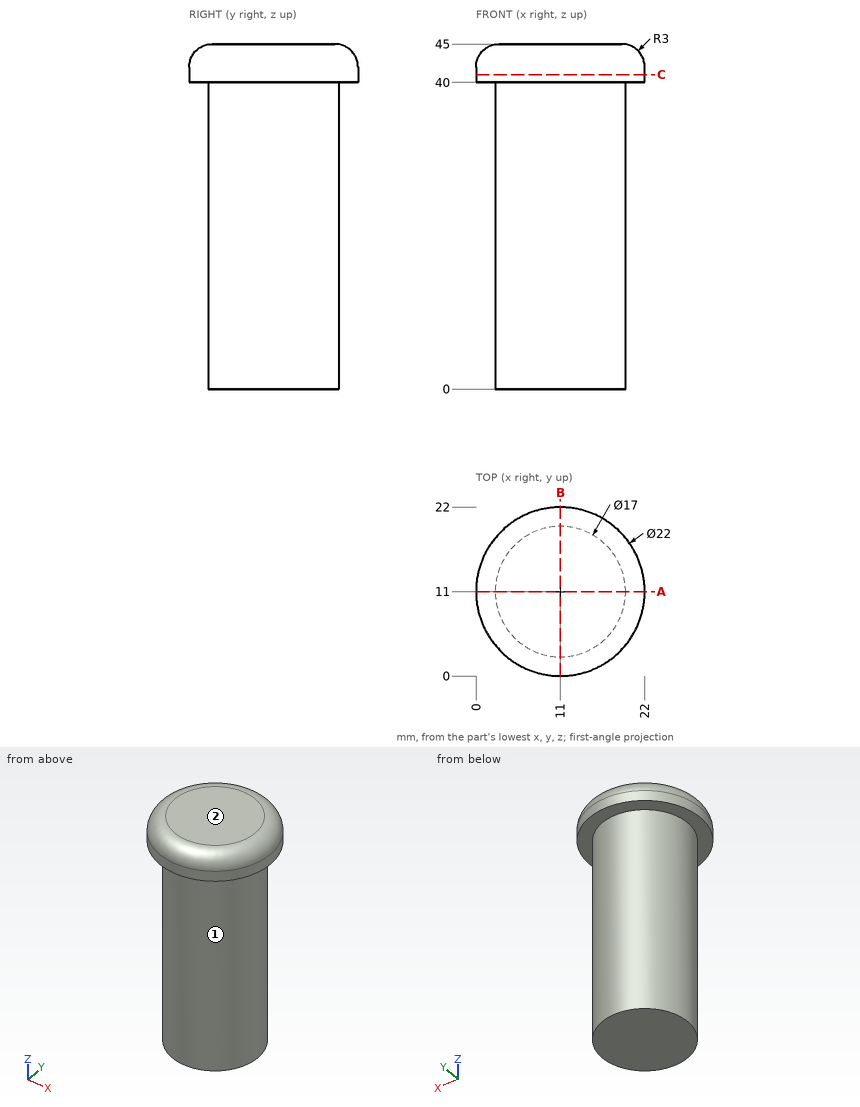
Job drawing, mm, ordinate dimensions from the low corner. One solid piece. A direction names the side the tool comes from. Coordinates: 2 decimals unless noted, no trailing zeros. Order: outer loops, then holes, each group sorted by start corner. A loop starts at its lowest first (then second) coordinate and runs counter-clockwise, first axis right, second up. Notation, with made-up numbers: (89, -29.5) - (105, -29.5) arc R24 ccw to (105, -19.5) - close; hole circle Ø1 at (75.5, -10). An arc over 180 degrees is marked (long way). Write each question's results on one line, items separated by ' | '. Start each with the question number.
Item 1: Wall check: probe 1 along Z at (x, y) = (9.5, 19); probe 2 along Z at (x, y) = (2, 11.25); probe 3 along Y at (x, z) = (10.75, 7). Give the ranges that are in metal, low to high. Write a range as [from, to].
Item 2: Band-saw the part on C-C on z = 41. Write the cut outline in (x, y).
Item 3: Band-saw the part on A-A on y = 11. Write the cut outline in (x, z), and give its area (3 significant figures).
Item 4: Flat gauge pins, fed straight in: pin 1 (2 mm diameter, centred on x = 19.5, z = 5, fed in from +Y); pin 2 (4 mm diameter, centred on x = 9, z = 29.5, fed in from -Y); pin 3 (1.5 mm diameter, centred on y = 3.5, z = 4.5, fed in from -X). Where does each tip first touch, or does it go through?
Item 5: Tool access for the marked faces 1 and 2: list every direction of +Z, -Z, +X, -X, +Y, -Y with a clear straight run to the whole face (end or side of a thin tool).
Numbers:
1) probe 1: [0, 45] | probe 2: [40, 44.83] | probe 3: [2.5, 19.5]
2) outline: circle Ø22 at (11, 11)
3) outline: (0, 40) - (2.5, 40) - (2.5, 0) - (19.5, 0) - (19.5, 40) - (22, 40) - (22, 42) arc R3 ccw to (19, 45) - (3, 45) arc R3 ccw to (0, 42) - close | area: 786 mm^2
4) pin 1: y = 15 | pin 2: y = 2.5 | pin 3: x = 5.83
5) face 1: -Z | face 2: +Z, +X, -X, +Y, -Y
